Here's how the part is built. I have some questions about the finished solid (model axes, mm). A direction names the side the tool comes from. Give positions to 0.01 mm unless a question says otherwise; leave off trailing zeros. Loops run counter-clockwise (first coordinate to the right, second up) from the corner with the lowest first, then second, coordinate; pieces in that order, holes last. Notation, with made-up numbers: (-11, 26.25) - (7, 26.25) arc R23 ccw to (7, 54.25) - close; hole circle Ø3 at (-15, -14.5). An arc over 180 degrees is marked (long way). One line per item, written item: value. Start each with the question number.
```python
from build123d import *

# Parameters (mm, degrees)
BOSS_EXTRUDE2_START     = -9.15
BOSS_EXTRUDE2_DEPTH     = 111.125
CUT_EXTRUDE2_DEPTH      = 53.975
SKETCH16_R              = 1.349999967
CUT_EXTRUDE3_DEPTH      = 112.125
CUT_EXTRUDE4_DEPTH      = 112.125000012
SKETCH22_R              = 1.849999983
CUT_EXTRUDE7_DEPTH      = 102.975000012
CUT_EXTRUDE7_DEPTH_BACK = 10.15
SKETCH23_W              = 28.575
SKETCH23_H              = 3.81
BOSS_EXTRUDE3_DEPTH     = 57.15
BOSS_EXTRUDE4_DEPTH     = 3.175
FILLET1_R               = 3.175
CUT_EXTRUDE8_DEPTH      = 112.125000012
CUT_EXTRUDE9_DEPTH      = 53.975
CUT_EXTRUDE12_DEPTH     = 82.55


with BuildPart() as part:
    # Sketch13 → Boss-Extrude2 (new body)
    with BuildSketch(Plane(origin=(0, 0, 0), x_dir=(1, 0, 0), z_dir=(0, 1, 0)).offset(BOSS_EXTRUDE2_START)):
        with BuildLine():
            Line((-51.435, -51.435), (0, -51.435))
            Line((0, -51.435), (0, -47.625))
            ThreePointArc((0, -47.625), (-12.296722124, -46.010121169), (-23.759524406, -41.275))
            Line((-23.759524406, -41.275), (-41.275, -41.275))
            Line((-41.275, -41.275), (-41.275, -23.759524406))
            ThreePointArc((-41.275, -23.759524406), (-47.625, 0), (-41.275, 23.759524406))
            Line((-41.275, 23.759524406), (-41.275, 41.275))
            Line((-41.275, 41.275), (-51.435, 51.435))
            Line((-51.435, 51.435), (-51.435, -51.435))
        make_face()
    boss_extrude2 = extrude(amount=BOSS_EXTRUDE2_DEPTH)

    # Sketch15 → Cut-Extrude2 (cut)
    with BuildSketch(Plane(origin=(0, 101.975000012, 0), x_dir=(1, 0, 0), z_dir=(0, 1, 0))):
        Polygon((0, 0), (-51.435, -51.435), (0, -51.435), align=None)
    cut_extrude2 = extrude(amount=-CUT_EXTRUDE2_DEPTH, mode=Mode.SUBTRACT)

    # Mirror1: Boss-Extrude2, Cut-Extrude2 across plane
    add(boss_extrude2.mirror(Plane(origin=(-51.435, 101.975000012, 51.435), x_dir=(0, 0, 1), z_dir=(1, 0, 0))))
    add(cut_extrude2.mirror(Plane(origin=(-51.435, 101.975000012, 51.435), x_dir=(0, 0, 1), z_dir=(1, 0, 0))), mode=Mode.SUBTRACT)

    # Sketch16 → Cut-Extrude3 (cut, through all)
    with BuildSketch(Plane.XZ.offset(9.149999988)):
        with Locations((-51.435, -13.335)):
            Circle(SKETCH16_R)
    extrude(amount=-CUT_EXTRUDE3_DEPTH, mode=Mode.SUBTRACT)

    # Sketch17 → Cut-Extrude4 (cut, through all)
    with BuildSketch(Plane(origin=(0, 101.975000012, 0), x_dir=(1, 0, 0), z_dir=(0, 1, 0))):
        Polygon((7.094402336, 7.094402336), (-7.094402336, -7.094402336), (-51.435, 37.246195329), (-95.775597664, -7.094402336), (-109.964402336, 7.094402336), (-58.529402336, 58.529402336), (-51.435, 51.435), (-44.340597664, 58.529402336), align=None)
    extrude(amount=-CUT_EXTRUDE4_DEPTH, mode=Mode.SUBTRACT)

    # Sketch22 → Cut-Extrude7 (cut, two sides)
    with BuildSketch(Plane(origin=(0, 0, 0), x_dir=(1, 0, 0), z_dir=(0, 1, 0))) as cut_extrude7_sk:
        with Locations((-51.435, -12.065)):
            Circle(SKETCH22_R)
    extrude(amount=CUT_EXTRUDE7_DEPTH, mode=Mode.SUBTRACT)
    extrude(cut_extrude7_sk.sketch, amount=-CUT_EXTRUDE7_DEPTH_BACK, mode=Mode.SUBTRACT)

    # Sketch23 → Boss-Extrude3 (add)
    with BuildSketch(Plane(origin=(0, 48.000000012, 0), x_dir=(1, 0, 0), z_dir=(0, 1, 0))):
        with Locations((14.2875, -49.53)):
            Rectangle(SKETCH23_W, SKETCH23_H)
        with Locations((-117.1575, -49.53)):
            Rectangle(SKETCH23_W, SKETCH23_H)
    extrude(amount=-BOSS_EXTRUDE3_DEPTH)

    # Sketch24 → Boss-Extrude4 (add)
    with BuildSketch(Plane(origin=(0, 48.000000012, 0), x_dir=(1, 0, 0), z_dir=(0, 1, 0))):
        with BuildLine():
            Line((28.575, -51.435), (-131.445, -51.435))
            ThreePointArc((-131.445, -51.435), (-51.435, -78.887051089), (28.575, -51.435))
        make_face()
    extrude(amount=-BOSS_EXTRUDE4_DEPTH)

    # Fillet1
    fillet1_edges = [part.edges().sort_by_distance(p)[0] for p in [
        (-117.1575, 48.000000012, 47.625),
        (-70.352737797, 48.000000012, 41.275),
        (-90.573277876, 48.000000012, 46.010121169),
    ]]
    fillet(fillet1_edges, radius=FILLET1_R)

    # Sketch25 → Cut-Extrude8 (cut, through all)
    with BuildSketch(Plane(origin=(0, 101.975000012, 0), x_dir=(1, 0, 0), z_dir=(0, 1, 0))):
        with BuildLine():
            Line((-58.42, -24.593444248), (-58.42, -39.959871939))
            Line((-58.42, -39.959871939), (-51.435, -46.944871939))
            Line((-51.435, -46.944871939), (-44.45, -39.959871939))
            Line((-44.45, -39.959871939), (-44.45, -24.593444248))
            ThreePointArc((-44.45, -24.593444248), (-46.543928705, -20.354427055), (-48.234688479, -15.939097443))
            ThreePointArc((-48.234688479, -15.939097443), (-51.435, -17.089999983), (-54.635311521, -15.939097443))
            ThreePointArc((-54.635311521, -15.939097443), (-56.326071295, -20.354427055), (-58.42, -24.593444248))
        make_face()
        with BuildLine():
            Line((-44.45, 25.771067268), (-44.45, 24.593444248))
            ThreePointArc((-44.45, 24.593444248), (-46.450454829, 20.566848232), (-48.087042692, 16.379142993))
            ThreePointArc((-48.087042692, 16.379142993), (-51.435, 17.859999967), (-54.782957308, 16.379142993))
            ThreePointArc((-54.782957308, 16.379142993), (-56.419545171, 20.566848232), (-58.42, 24.593444248))
            Line((-58.42, 24.593444248), (-58.42, 25.771067268))
            Line((-58.42, 25.771067268), (-51.435, 32.756067268))
            Line((-51.435, 32.756067268), (-44.45, 25.771067268))
        make_face()
    extrude(amount=-CUT_EXTRUDE8_DEPTH, mode=Mode.SUBTRACT)

    # Sketch26 → Cut-Extrude9 (cut)
    with BuildSketch(Plane.XZ.offset(9.149999988)):
        with BuildLine():
            Line((-44.45, 44.45), (-48.26, 48.26))
            Line((-48.26, 48.26), (-15.862294916, 48.26))
            ThreePointArc((-15.862294916, 48.26), (-20.317375146, 46.560114553), (-24.593444248, 44.45))
            Line((-24.593444248, 44.45), (-44.45, 44.45))
        make_face()
        with BuildLine():
            Line((-58.42, 44.45), (-54.61, 48.26))
            Line((-54.61, 48.26), (-87.007705084, 48.26))
            ThreePointArc((-87.007705084, 48.26), (-82.552624854, 46.560114553), (-78.276555752, 44.45))
            Line((-78.276555752, 44.45), (-58.42, 44.45))
        make_face()
    extrude(amount=-CUT_EXTRUDE9_DEPTH, mode=Mode.SUBTRACT)

    # Sketch30 → Cut-Extrude12 (cut)
    with BuildSketch(Plane(origin=(0, 101.975000012, 0), x_dir=(1, 0, 0), z_dir=(0, 1, 0))):
        with BuildLine():
            Line((-44.45, 25.771067268), (-51.435, 32.756067268))
            Line((-51.435, 32.756067268), (-58.42, 25.771067268))
            Line((-58.42, 25.771067268), (-58.42, 24.593444248))
            ThreePointArc((-58.42, 24.593444248), (-52.07, 0), (-58.42, -24.593444248))
            Line((-58.42, -24.593444248), (-58.42, -39.959871939))
            Line((-58.42, -39.959871939), (-51.435, -46.944871939))
            Line((-51.435, -46.944871939), (-44.45, -39.959871939))
            Line((-44.45, -39.959871939), (-44.45, -24.593444248))
            ThreePointArc((-44.45, -24.593444248), (-50.8, 0), (-44.45, 24.593444248))
            Line((-44.45, 24.593444248), (-44.45, 25.771067268))
        make_face()
    extrude(amount=-CUT_EXTRUDE12_DEPTH, mode=Mode.SUBTRACT)


solid = part.part
```
(1) If we section it at C-C on x = -66.5: List the corners of the cut face in (y, z) for me (3 decimals), plus the area to 3 significant figures.
(2) If we section it at D-D on z = -5: List the corners of the cut face in (x, y) for me (3 decimals), plus the area to 3 significant figures.
(3) Will these pins go through, and if not, where does the flat tip stop? pin 1 (14.5 mm diameter, centred on x = 12, y = 28, fed in from -Z) (3 decimals); pin 2 (4 mm diameter, centred on x = -113, y = 42.5, fed in from +Z) (3 decimals); pin 3 (10 mm diameter, centred on y = 47, z = 28.5, fed in from -X) (3 decimals); pin 4 (12 mm diameter, centred on y = 66.5, z = 59.5, fed in from -X).
(4) For faces 5 (the face through (-51, 19.425, -1)), 6 (the face through (-47.99, 47.19, 43.5)), 7 (the face through (-70, 17, 41.275)), 8 (the face through (-68, 17, 44.45)), 9 (the face through (-32, 19, 41.275)), which set-ups out of +Z, -Z, +X, -X, +Y, -Y let a thin tool reach every point of the face, with its end or its side?
(5) If we mould it in two halves opening along Z, with no side actions, what happens to faces 1 (the face through (-41.275, 46, 33)), 2 (the face through (-12.128, 19.025, 46.055)), 3 (the face through (-46, 17, 46)), 4 (the face through (-58.42, 47, 32))? For each: pulls with the +Z half, pulls with the -Z half, needs draft (parallel to the pull), parting line crosses it, or undercut.
(6) If we section it at B-B on z = 32: List the corners of the cut face in (x, y) for me (3 decimals), plus the area to 3 significant figures.
(7) Please list where these lines run through material, in increasing order: probe 1 along X at (y, z) = (80.5, 40) (3 decimals); probe 2 along Z at (x, y) = (-43, -2) (3 decimals); probe 3 along Z at (x, y) = (-31.5, 7) (3 decimals). Write a range as from..to.
(8) If we section it at A-A on y = 90: List the corners of the cut face in (x, z) for me (3 decimals), plus the area to 3 significant figures.
Found:
1. outline: (-9.15, 41.275) - (44.825, 41.275) arc R3.175 ccw to (48, 44.45) - (48, 78.013) - (44.825, 78.013) - (44.825, 51.435) - (-9.15, 51.435) - (-9.15, 48.26) - (44.825, 48.26) - (44.825, 44.45) - (-9.15, 44.45) - close
1. area: 457 mm^2
2. outline: (-55.508, -9.15) - (-47.362, -9.15) - (-47.362, 101.975) - (-50.553, 101.975) - (-50.553, 19.425) - (-52.317, 19.425) - (-52.317, 101.975) - (-55.508, 101.975) - close
2. area: 760 mm^2
3. pin 1: z = 47.625
3. pin 2: z = 51.435
3. pin 3: x = -61.595
3. pin 4: through
4. face 5: +Y
4. face 6: +Y, -Y
4. face 7: -Z, -X, +Y, -Y
4. face 8: -Y
4. face 9: -Z, +X, +Y, -Y
5. face 1: needs draft
5. face 2: pulls with the -Z half
5. face 3: undercut
5. face 4: undercut
6. outline: (-61.595, -9.15) - (-58.42, -9.15) - (-58.42, 101.975) - (-61.595, 101.975) - close; (-44.45, -9.15) - (-41.275, -9.15) - (-41.275, 101.975) - (-44.45, 101.975) - close
6. area: 706 mm^2
7. probe 1: -61.595..-58.38, -44.49..-41.275
7. probe 2: -28.811..-20.473, 20.473..44.45, 48.26..51.435
7. probe 3: 41.275..44.45, 48.26..51.435
8. outline: (-61.595, -27.086) - (-51.435, -37.246) - (-41.275, -27.086) - (-41.275, -23.76) arc R47.625 cw to (-41.275, 23.76) - (-41.275, 41.275) - (-51.435, 51.435) - (-61.595, 41.275) - (-61.595, 23.76) arc R47.625 cw to (-61.595, -23.76) - close; hole (-58.42, -25.771) - (-51.435, -32.756) - (-44.45, -25.771) - (-44.45, -24.593) arc R50.8 cw to (-44.45, 24.593) - (-44.45, 39.96) - (-51.435, 46.945) - (-58.42, 39.96) - (-58.42, 24.593) arc R50.8 cw to (-58.42, -24.593) - close
8. area: 594 mm^2
